Check sheet for the modelled part. Datum: model origin and axes. Units: mm. Face numbers are marked on the shaded views. A direction names the side the tool comes from. Round coordinates to 2 decimals unless told otherwise and drop trailing zeros. Write each loop counter-clockwise with the first axis right and the second up, starting at its lowest first coordinate (ties: lowest second). Pieces come first, ordered by that corner, then holes.
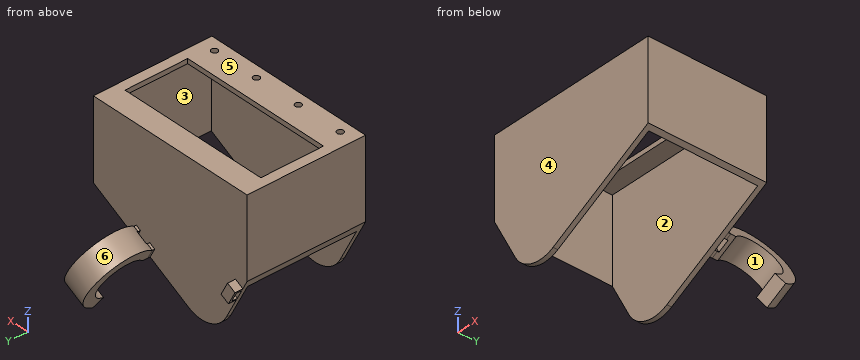
from build123d import *

# Parameters (mm, degrees)
RESSALTO_EXTRUS_O4_DEPTH  = 75
CASCA4_T                  = -3
ESBO_O13_R                = 2
ESBO_O13_W                = 97.172868657
ESBO_O13_H                = 39.686100031
CORTE_EXTRUS_O2_DEPTH     = 75
RESSALTO_EXTRUS_O7_DEPTH  = 5
ESBO_O21_W                = 7
ESBO_O21_H                = 3.5
CORTE_EXTRUS_O7_DEPTH     = 15
RESSALTO_EXTRUS_O9_DEPTH  = 1.5
RESSALTO_EXTRUS_O10_DEPTH = 15
CORTE_EXTRUS_O8_DEPTH     = 9


with BuildPart() as part:
    # Esboço1 → Ressalto-extrusão4 (new body)
    with BuildSketch(Plane(origin=(0, 0, 0), x_dir=(1, 0, 0), z_dir=(0, 1, 0))):
        with BuildLine():
            Line((-61.526708671, 22.298270257), (-61.526708671, -27.701729743))
            Line((-61.526708671, -27.701729743), (48.473291329, -27.701729743))
            Line((48.473291329, -27.701729743), (48.473291329, 22.462720238))
            Line((48.473291329, 22.462720238), (-19.533044421, 58.851024019))
            ThreePointArc((-19.533044421, 58.851024019), (-34.831371888, 60.338136116), (-46.667038922, 50.53164278))
            Line((-46.667038922, 50.53164278), (-61.526708671, 22.298270257))
        make_face()
    extrude(amount=RESSALTO_EXTRUS_O4_DEPTH)

    # Casca4
    casca4_openings = [part.faces().sort_by_distance(p)[0] for p in [
        (-34.831371888, 37.5, -60.338136116),
        (14.470123454, 37.5, -40.656872128),
        (-54.096873797, 37.5, -36.414956518),
    ]]
    offset(amount=CASCA4_T, openings=casca4_openings, kind=Kind.INTERSECTION)

    # Esboço13 → Corte-extrusão2 (cut)
    with BuildSketch(Plane.XY.offset(27.701729743)):
        with Locations((8.473291329, 7.143908188)):
            Circle(ESBO_O13_R)
        with Locations((38.473291329, 7.143908188)):
            Circle(ESBO_O13_R)
        with Locations(Location((-51.526708671, 7.143908188, 0), (0, 0, 180))):
            Circle(ESBO_O13_R)
        with Locations(Location((-21.526708671, 7.143908188, 0), (0, 0, 180))):
            Circle(ESBO_O13_R)
        with Locations((-6.526708671, 40.786037138)):
            Rectangle(ESBO_O13_W, ESBO_O13_H)
    extrude(amount=-CORTE_EXTRUS_O2_DEPTH, mode=Mode.SUBTRACT)

    # Esboço20 → Ressalto-extrusão7 (add)
    with BuildSketch(Plane(origin=(0, 75, 0), x_dir=(1, 0, 0), z_dir=(0, 1, 0))):
        Polygon((-48.559735009, 34.052973883), (-53.869244343, 36.84745248), (-58.526708671, 27.998270257), (-53.217199337, 25.20379166), align=None)
    extrude(amount=RESSALTO_EXTRUS_O7_DEPTH)

    # Esboço21 → Corte-extrusão7 (cut)
    with BuildSketch(Plane(origin=(-52.061018169, 0, -27.400535878), x_dir=(0.46574643283262207, 0, -0.8849182223819825), z_dir=(0.8849182223819825, 0, 0.46574643283262207))):
        with Locations((2.517573756, 76.75)):
            Rectangle(ESBO_O21_W, ESBO_O21_H)
    extrude(amount=-CORTE_EXTRUS_O7_DEPTH, mode=Mode.SUBTRACT)

    # Esboço23 → Ressalto-extrusão9 (add)
    with BuildSketch(Plane(origin=(0, 75, 0), x_dir=(1, 0, 0), z_dir=(0, 1, 0))):
        Polygon((17.78051848, 30.946502751), (21.082988999, 37.118511214), (14.470123454, 40.656872128), (7.857257909, 44.195233042), (4.55478739, 38.023224579), align=None)
    extrude(amount=RESSALTO_EXTRUS_O9_DEPTH)

    # Esboço27 → Ressalto-extrusão10 (add)
    with BuildSketch(Plane(origin=(0.949934773, 0, 0.508283746), x_dir=(0.4717815026852956, 0, -0.8817154947736852), z_dir=(0.8817154947736852, 0, 0.4717815026852957))):
        with BuildLine():
            Line((42.674530712, 76.5), (42.674530712, 79.859907211))
            ThreePointArc((42.674530712, 79.859907211), (43.504490054, 102.339384634), (64.83991575, 95.21089615))
            Line((64.83991575, 95.21089615), (70.983567604, 99.465779677))
            ThreePointArc((70.983567604, 99.465779677), (39.876872471, 108.665113983), (35.674530712, 76.5))
            Line((35.674530712, 76.5), (42.674530712, 76.5))
        make_face()
    extrude(amount=-RESSALTO_EXTRUS_O10_DEPTH)

    # Esboço28 → Corte-extrusão8 (cut)
    with BuildSketch(Plane(origin=(20.133054226, 0, -37.626794961), x_dir=(-0.8817154947736852, 0, -0.4717815026852955), z_dir=(0.4717815026852955, 0, -0.8817154947736852))):
        Polygon((2.309694071, 75), (2.309694071, 77.5), (9.809694071, 77.5), (9.809694071, 75), (6.059694071, 75), align=None)
    extrude(amount=-CORTE_EXTRUS_O8_DEPTH, mode=Mode.SUBTRACT)


solid = part.part
1. Sectioned sample at D-D, the plane y = 97. Enter the section's corners in (x, z), plus the area to 3 significant figures.
2. Sectioned sample at B-B, the plane z = 9. Enter the section's corners in (x, y), plus the area to 3 significant figures.
3. Release check for a two-part mould opening along Y. For the marked faces 3, 4, 5 and 6 record: released by +Y, released by -Y, zero draft, split by the parting line, or undercut.
4. Go/stop test with flat-tipped pins: pin 1 (2 mm diameter, centred on x = 23.5, z = 4, fed in from +Y); pin 2 (1.5 mm diameter, centred on x = 31, z = -58, fed in from +Y); pin 3 (11 mm diameter, centred on x = -56, z = -31.5, fed in from +Y). Record where each tip stops, or that it passes through.
5. Scan lines: line 1 along Y through (x, z) = (-18, -8); line 2 along Y through (x, z) = (19, -36); line 3 along X through (y, z) = (59.5, -20). Record each from-to range of solid material in increasing order.
6. Sectioned sample at A-A, the plane y = 31.5. Enter the section's corners in (x, z).
7. Set-up check for the marked faces 1 and 2: record each of +Z, -Z, +X, -X, +Y, -Y from which the full face is reachable in a straight line by a thin tool's end or side.
8. Sectioned sample at C-C, the plane x = -7.5. Enter the section's corners in (y, z).
Computed values:
1. outline: (2.4, -33.99) - (6.08, -40.87) - (19.3, -33.79) - (15.62, -26.92) - close; (17.97, -63.09) - (19.53, -66.02) - (32.76, -58.94) - (31.19, -56.02) - close
1. area: 167 mm2
2. outline: (-61.53, 0) - (48.47, 0) - (48.47, 75) - (-61.53, 75) - close; hole (-58.53, 3) - (45.47, 3) - (45.47, 72) - (-58.53, 72) - close
2. area: 1,070 mm2
3. face 3: undercut
3. face 4: released by -Y
3. face 5: zero draft
3. face 6: undercut
4. pin 1: stops at y = 75
4. pin 2: stops at y = 107.29
4. pin 3: stops at y = 80
5. line 1: y = 0 to 3, 72 to 75
5. line 2: y = 0 to 3, 72 to 81.8, 99.78 to 109.18
5. line 3: x = -61.53 to -58.53, 45.47 to 48.47
6. outline: (-61.53, -22.3) - (-58.53, -28) - (-58.53, 24.7) - (-55.11, 24.7) - (-55.11, 27.7) - (-61.53, 27.7) - close; (42.06, 24.7) - (45.47, 24.7) - (45.47, -24.07) - (48.47, -22.46) - (48.47, 27.7) - (42.06, 27.7) - close
7. face 1: none
7. face 2: -Z
8. outline: (0, -52.41) - (3, -52.41) - (3, 24.7) - (20.94, 24.7) - (20.94, 27.7) - (0, 27.7) - close; (60.63, 24.7) - (72, 24.7) - (72, -52.41) - (75, -52.41) - (75, 27.7) - (60.63, 27.7) - close
